Build history of the part. All positions in model axes, mm. A direction names the side the tool comes from. Round coordinates to 2 decimals unless told otherwise and drop trailing zeros. Write each loop counter-clockwise with the first axis right and the second up, starting at its lowest first coordinate (ties: lowest second). Pieces come first, ordered by that corner, then holes. Notation, with made-up numbers: (52, -24.75) -> (70, -24.75) arc R33 cw to (70, 6.25) -> close; hole circle Ø7 at (-33.5, -16). An arc over 180 degrees is marked (long way). Answer as CSV lines item,"result".
from build123d import *

# Parameters (mm, degrees)
BOSS_EXTRUDE1_DEPTH = 3.175
CUT_EXTRUDE1_DEPTH  = 204.138678001
SKETCH3_W           = 42
SKETCH3_H           = 55.35
SKETCH3_W_2         = 7.65
SKETCH3_H_2         = 6.35
CUT_EXTRUDE2_DEPTH  = 204.138678001
FILLET3_R           = 5
SKETCH5_R           = 2
CUT_EXTRUDE4_DEPTH  = 204.138678001
CUT_EXTRUDE5_DEPTH  = 204.138678001
FILLET5_R           = 76
FILLET6_R           = 7


with BuildPart() as part:
    # Sketch1 → Boss-Extrude1 (new, symmetric)
    with BuildSketch(Plane(origin=(0, 0, 0), x_dir=(1, 0, 0), z_dir=(0, 1, 0))):
        with BuildLine():
            Line((35, -200), (35, 0))
            ThreePointArc((35, 0), (0, 35), (-35, 0))
            Line((-35, 0), (-35, -200))
            Line((-35, -200), (35, -200))
        make_face()
    extrude(amount=BOSS_EXTRUDE1_DEPTH, both=True)

    # Sketch2 → Cut-Extrude1 (cut, through all)
    with BuildSketch(Plane(origin=(0, 3.175, 0), x_dir=(1, 0, 0), z_dir=(0, 1, 0))):
        with BuildLine():
            Line((-35, -38), (35, -38))
            Line((35, -38), (35, 0))
            ThreePointArc((35, 0), (0, 35), (-35, 0))
            Line((-35, 0), (-35, -38))
        make_face()
    extrude(amount=-CUT_EXTRUDE1_DEPTH, mode=Mode.SUBTRACT)

    # Sketch3 → Cut-Extrude2 (cut, through all)
    with BuildSketch(Plane(origin=(0, 3.175, 0), x_dir=(1, 0, 0), z_dir=(0, 1, 0))):
        with Locations((0, -162.325)):
            Rectangle(SKETCH3_W, SKETCH3_H)
        with Locations((-24.825, -186.825)):
            Rectangle(SKETCH3_W_2, SKETCH3_H_2)
        with Locations((24.825, -186.825)):
            Rectangle(SKETCH3_W_2, SKETCH3_H_2)
    extrude(amount=-CUT_EXTRUDE2_DEPTH, mode=Mode.SUBTRACT)

    # Fillet3
    fillet3_edges = [part.edges().sort_by_distance(p)[0] for p in [
        (35, 0, 200),
        (-35, 0, 200),
    ]]
    fillet(fillet3_edges, radius=FILLET3_R)

    # Sketch5 → Cut-Extrude4 (cut, through all)
    with BuildSketch(Plane(origin=(0, 3.175, 0), x_dir=(1, 0, 0), z_dir=(0, 1, 0))):
        with Locations(Location((27.5, -195.35, 0), (0, 0, 270))):
            Circle(SKETCH5_R)
        with Locations(Location((-27.5, -195.35, 0), (0, 0, 270))):
            Circle(SKETCH5_R)
        with Locations(Location((15, -65.35, 0), (0, 0, 270))):
            Circle(SKETCH5_R)
        with Locations(Location((-15, -65.35, 0), (0, 0, 270))):
            Circle(SKETCH5_R)
    extrude(amount=-CUT_EXTRUDE4_DEPTH, mode=Mode.SUBTRACT)

    # Sketch6 → Cut-Extrude5 (cut, through all)
    with BuildSketch(Plane(origin=(0, 3.175, 0), x_dir=(1, 0, 0), z_dir=(0, 1, 0))):
        with BuildLine():
            Line((-35, -134.65), (-35, -49.65))
            ThreePointArc((-35, -49.65), (-18.102907984, -92.15), (-35, -134.65))
        make_face()
    cut_extrude5 = extrude(amount=-CUT_EXTRUDE5_DEPTH, mode=Mode.SUBTRACT)

    # Mirror1: Cut-Extrude5 across plane
    add(cut_extrude5.mirror(Plane(origin=(0, 0, 0), x_dir=(0, 0, 1), z_dir=(1, 0, 0))), mode=Mode.SUBTRACT)

    # Fillet5
    # the kernel refuses this fillet: 76 mm, written as the material it takes off along each edge
    with BuildSketch(Plane(origin=(-35, 39.601520625, 49.65), x_dir=(0, 0, -1), z_dir=(0, -1, 0))) as fillet5_piece_1:
        with BuildLine():
            CenterArc((26.124451555, 74.608915367), FILLET5_R, 240.155370723, 18.865389254)
            Line((-11.696928446, 8.688181035), (-12.453356046, 7.369766348))
            ThreePointArc((-12.453356046, 7.369766348), (-6.498269887, 3.469254885), (-1.04366777, -1.105059992))
            Line((-1.04366777, -1.105059992), (0, -1.52))
            ThreePointArc((0, -1.52), (5.825, -1.52), (11.360510969, -1.492178307))
            Line((11.360510969, -1.492178307), (11.65, 0))
        make_face()
    extrude(amount=79.20304125, mode=Mode.SUBTRACT)
    with BuildSketch(Plane(origin=(-35, 62.277048415, 134.65), x_dir=(0.587963491001448, 0, -0.8088874663693276), z_dir=(0, -1, 0))) as fillet5_piece_2:
        with BuildLine():
            CenterArc((25.562462836, 75.375386129), FILLET5_R, 233.987375861, 28.66182532)
            Line((-19.12276248, 13.899938684), (-20.016466986, 12.670429736))
            Line((-20.016466986, 12.670429736), (-0.893704506, -1.229508949))
            Line((-0.893704506, -1.229508949), (0.194474848, -1.507507723))
            ThreePointArc((0.194474848, -1.507507723), (7.919360226, -1.011292338), (15.644245604, -1.507507723))
            Line((15.644245604, -1.507507723), (15.838720451, 0))
        make_face()
    extrude(amount=124.554096829, mode=Mode.SUBTRACT)
    with BuildSketch(Plane(origin=(35, 62.277048415, 134.65), x_dir=(-0.587963491001448, 0, -0.8088874663693276), z_dir=(0, -1, 0))) as fillet5_piece_3:
        with BuildLine():
            CenterArc((25.562462836, -75.375386129), FILLET5_R, 97.350798819, 28.66182532)
            Line((-19.12276248, -13.899938684), (-20.016466986, -12.670429736))
            Line((-20.016466986, -12.670429736), (-0.893704506, 1.229508949))
            Line((-0.893704506, 1.229508949), (0.194474848, 1.507507723))
            ThreePointArc((0.194474848, 1.507507723), (7.919360226, 1.011292338), (15.644245604, 1.507507723))
            Line((15.644245604, 1.507507723), (15.838720451, 0))
        make_face()
    extrude(amount=124.554096829, mode=Mode.SUBTRACT)
    with BuildSketch(Plane(origin=(35, 39.601520625, 49.65), x_dir=(0, 0, -1), z_dir=(0, -1, 0))) as fillet5_piece_4:
        with BuildLine():
            CenterArc((26.124451555, -74.608915367), FILLET5_R, 100.979240023, 18.865389254)
            Line((-11.696928446, -8.688181035), (-12.453356046, -7.369766348))
            ThreePointArc((-12.453356046, -7.369766348), (-6.498269887, -3.469254885), (-1.04366777, 1.105059992))
            Line((-1.04366777, 1.105059992), (0, 1.52))
            ThreePointArc((0, 1.52), (5.825, 1.52), (11.360510969, 1.492178307))
            Line((11.360510969, 1.492178307), (11.65, 0))
        make_face()
    extrude(amount=79.20304125, mode=Mode.SUBTRACT)

    # Fillet6
    fillet6_edges = [part.edges().sort_by_distance(p)[0] for p in [
        (35, 0, 38),
        (-35, 0, 38),
    ]]
    fillet(fillet6_edges, radius=FILLET6_R)


solid = part.part
1. Which spindle directions (+Z, -Z, +X, -X, +Y, -Y) get a long thin tool onto all of the face, cutting with end or side? Do faces 4 (the flat face through (28.65, 0, 187)), 5 (the cylindrical face through (-29.782, 0.044, 54.523)), 6 (the flat face through (35, 0, 177)), 7 (the flat face through (0, 0, 200)), 8 (the cylindrical face through (32.57, 0.04, 139.22)). Say none if no direction does.
Results found:
face 4,"+Y, -Y"
face 5,"-X, +Y, -Y"
face 6,"+Z, -Z, +X, +Y, -Y"
face 7,"+Z, +X, -X, +Y, -Y"
face 8,"+X, +Y, -Y"
2. Drop flat-ended pins along their axis: pin 1 Ø1.5 at (y, z) = (-2, 128.5) entering from -X; pin 2 Ø12 at (x, z) = (-14.5, 169.5) entering from -Y. Give the stop position or say it passes through.
Results found:
pin 1,"stops at x = -29.23"
pin 2,"passes through"
3. Cut at B-B, the plane z = 186. Write the cut outline in (x, y) (3 decimals).
Results found:
outline,"(-35, -3.175) -> (-28.65, -3.175) -> (-28.65, 3.175) -> (-35, 3.175) -> close; (28.65, -3.175) -> (35, -3.175) -> (35, 3.175) -> (28.65, 3.175) -> close"
4. Cut at C-C, the plane x = -15. Write the cut outline in (y, z) (3 decimals).
Results found:
outline,"(-3.175, 38) -> (3.175, 38) -> (3.175, 63.35) -> (-3.175, 63.35) -> close; (-3.175, 67.35) -> (3.175, 67.35) -> (3.175, 134.65) -> (-3.175, 134.65) -> close; (-3.175, 190) -> (3.175, 190) -> (3.175, 200) -> (-3.175, 200) -> close"
5. Probe line 1 along X through (y, z) = (-0.75, 195.35); line 2 along Z through (x, y) = (28.5, -1); line 3 along Z through (x, y) = (-3.5, -0.25). List the from-to ranges inside material, lowest first.
Results found:
line 1,"x = -34.99 to -29.5, -25.5 to 25.5, 29.5 to 34.99"
line 2,"z = 38.48 to 57.25, 127.54 to 183.65, 190 to 193.62, 197.08 to 200"
line 3,"z = 38 to 134.65, 190 to 200"
6. Cut at A-A, the plane x = 0.5. Write the cut outline in (y, z) (3 decimals), then the cut area to 3 significant figures.
Results found:
outline,"(-3.175, 38) -> (3.175, 38) -> (3.175, 134.65) -> (-3.175, 134.65) -> close; (-3.175, 190) -> (3.175, 190) -> (3.175, 200) -> (-3.175, 200) -> close"
area,"677 mm2"
7. Mould opens along X. For faces 1 (the flat face through (-28.65, 0, 187)), 2 (the flat face through (-35, 0, 176)), 3 (the flat face through (0, 3.175, 100)) say: +X half, -X half, draft (parallel to the pull), parting line (faces both ways), or undercut.
Results found:
face 1,"undercut"
face 2,"-X half"
face 3,"draft"
8. Cut at D-D, the plane y = 2. Write the cut outline in (x, z), then the cut area to 3 significant figures.
Results found:
outline,"(-35, 158.29) arc R76 ccw to (-25.69, 121.84) arc R61.9 cw to (-26.31, 61.35) arc R76 ccw to (-32.62, 47.18) arc R7 ccw to (-25.96, 38) -> (25.96, 38) arc R7 ccw to (32.62, 47.18) arc R76 ccw to (26.31, 61.35) arc R61.9 cw to (25.69, 121.84) arc R76 ccw to (35, 158.29) -> (35, 195) arc R5 ccw to (30, 200) -> (-30, 200) arc R5 ccw to (-35, 195) -> close; hole circle Ø4 at (-27.5, 195.35); hole (-28.65, 183.65) -> (-21, 183.65) -> (-21, 134.65) -> (21, 134.65) -> (21, 183.65) -> (28.65, 183.65) -> (28.65, 190) -> (-28.65, 190) -> close; hole circle Ø4 at (-15, 65.35); hole circle Ø4 at (15, 65.35); hole circle Ø4 at (27.5, 195.35)"
area,"6,690 mm2"
